from build123d import *

# Parameters (mm, degrees)
ESQUISSE1_R             = 19.05
BOSS_EXTRU_1_DEPTH      = 2.032
ESQUISSE2_R             = 11.811
BOSS_EXTRU_2_DEPTH      = 5.08
ESQUISSE3_R             = 5.0165
ENL_V_MAT_EXTRU_1_DEPTH = 1.524
ESQUISSE4_R             = 7.875
BOSS_EXTRU_3_DEPTH      = 9
ESQUISSE5_R             = 6.875
ENL_V_MAT_EXTRU_2_DEPTH = 14.588


with BuildPart() as part:
    # Esquisse1 → Boss.-Extru.1 (new body)
    with BuildSketch(Plane.XY):
        Circle(ESQUISSE1_R)
    extrude(amount=BOSS_EXTRU_1_DEPTH)

    # Esquisse2 → Boss.-Extru.2 (add)
    with BuildSketch(Plane.XY.offset(2.032)):
        Circle(ESQUISSE2_R)
    extrude(amount=BOSS_EXTRU_2_DEPTH)

    # Esquisse3 → Enlèv. mat.-Extru.1 (cut)
    with BuildSketch(Plane.XY.offset(7.112)):
        Circle(ESQUISSE3_R)
    extrude(amount=-ENL_V_MAT_EXTRU_1_DEPTH, mode=Mode.SUBTRACT)

    # Esquisse4 → Boss.-Extru.3 (add)
    with BuildSketch(Plane(origin=(0, 0, 0), x_dir=(-1, 0, 0), z_dir=(0, 0, -1))):
        with Locations(Location((0, 0, 0), (0, 0, 180))):
            Circle(ESQUISSE4_R)
    extrude(amount=BOSS_EXTRU_3_DEPTH)

    # Esquisse5 → Enlèv. mat.-Extru.2 (cut)
    with BuildSketch(Plane(origin=(0, 0, -9), x_dir=(-1, 0, 0), z_dir=(0, 0, -1))):
        Circle(ESQUISSE5_R)
    extrude(amount=-ENL_V_MAT_EXTRU_2_DEPTH, mode=Mode.SUBTRACT)


solid = part.part
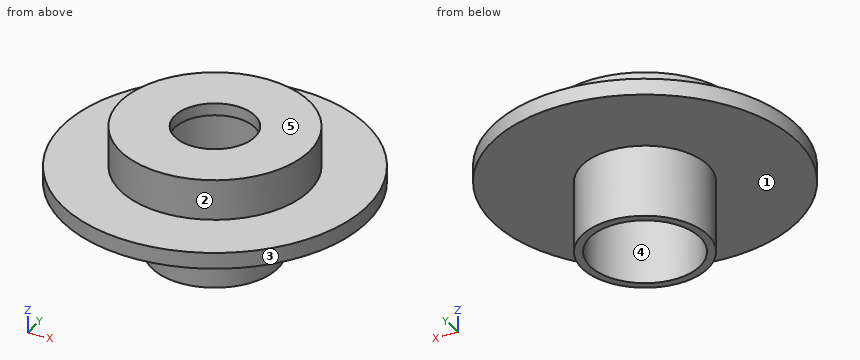
Work out the finished part from the listing and answer in its coordinate system (mm). Face numbers are marked on the shaded views. A direction names the side the tool comes from. Give positions to 0.01 mm unless a question says otherwise; leave off trailing zeros. Order: outer loops, then holes, each group sorted by start corner. A loop starts at its lowest first (then second) coordinate and runs counter-clockwise, first axis right, second up. Notation, with made-up numbers: (48, 20) -> (79, 20) arc R14 ccw to (79, 26) -> close; hole circle Ø7 at (17, 62.5). An arc over 180 degrees is marked (long way). Answer as a JSON object with one key per item and string values. Group by question number.
1. A tool of negligible diameter and unlimited length cuts with its end or side. For the marked faces 1 and 2, from which of +Z, -Z, +X, -X, +Y, -Y can it reach the whole face along a straight path? Write none if from no direction.
2. Flat-ended cylindrical pins translate along their axes: pin 1 Ø11.5 at (x, y) = (0, 0) entering from -Z; pin 2 Ø8 at (x, y) = (2.5, -8.5) entering from -Z; pin 3 Ø4 at (x, y) = (13.5, 11.5) entering from -Z; pin 4 Ø5 at (x, z) = (-11, 5.5) entering from -Y. Find the tip coordinate at first contact, or state that the pin passes through.
3. Section D-D on x = -9 is taken. Determine the outline of the cut face in (y, z), plus the area to 3 significant figures.
4. Section C-C on z = -6 is taken. Determine the outline of the cut face in (x, y) (3 decimals), plus the area to 3 significant figures.
5. Consider line 1 along Y through (x, z) = (0, -1.5) (3 decimals); line 2 along Z through (x, y) = (-1, 9); line 3 along Z through (x, y) = (3, 5.5). Determine where each line is inside the solid, lowest interval first. Write a range as [from, to].
6. The mould has two halves that part along X. Classify the marked faces 3, 4 and 5: released by +X, released by -X, zero draft, split by the parting line, or undercut.
Result sheet:
{
 "1": {"face 1": "-Z", "face 2": "+Z"},
 "2": {"pin 1": "stops at z = 5.59", "pin 2": "stops at z = -9", "pin 3": "stops at z = 0", "pin 4": "stops at y = -8.2"},
 "3": {"outline": "(-16.79, 0) -> (16.79, 0) -> (16.79, 2.03) -> (7.65, 2.03) -> (7.65, 7.11) -> (-7.65, 7.11) -> (-7.65, 2.03) -> (-16.79, 2.03) -> close", "area": "146 mm^2"},
 "4": {"outline": "circle Ø15.75 at (0, 0); hole circle Ø13.75 at (0, 0)", "area": "46.3 mm^2"},
 "5": {"line 1": "y = [-7.875, -6.875], [6.875, 7.875]", "line 2": "z = [0, 7.11]", "line 3": "z = [5.59, 7.11]"},
 "6": {"face 3": "split by the parting line", "face 4": "undercut", "face 5": "zero draft"}
}
